Input: part model. Units: mm. Frame: model coordinates. A direction names the side the tool comes from. Give positions to 0.01 mm unless a question says otherwise; leave off trailing zeros. Loops run counter-clockwise (first coordinate to the right, second up) from the corner with the lowest first, then second, coordinate; pieces in that order, holes last. Notation, with made-up numbers: M -26,83 L 16,83 A3 cw 16,88 Z; hole C 86.25,28.25 d9. An arc over 180 degrees is marked long. One line per item, written item: value. Start each with the question number.
(1) Access query for faces 1 (the flat face through (0, 15, -26)), 2 (the flat face through (60, 15, -26)), 3 (the flat face through (30, 23.8, -6)), 4 (the flat face through (-23.293, 32, -27)), 5 (the flat face through (35, 31.5, -34)). Directions: +Z, -Z, +X, -X, +Y, -Y. A direction counts if a zero-diameter tool reaches every point of the face in a straight line with its end or side. Return the directions, or none.
(2) Section C-C on x = -6. Output: boundary loops of the cut face in (y, z), plus the area to 3 significant figures.
(3) Section B-B on z = -18. Output: boundary loops of the cut face in (x, y).
(4) Section A-A on y = 28. Output: boundary loops of the cut face in (x, z) (3 decimals), plus the area to 3 significant figures.
(5) Section D-D on y = 22. Output: boundary loops of the cut face in (x, z) (3 decimals), plus the area to 3 significant figures.
(6) Pull-direction query (Y, two-part tool) for faces 6 (the flat face through (30, 7.4, -6)), 7 (the flat face through (31, 34.5, -27)), 8 (the cylindrical face through (35.243, 15.971, -18.54)); classes: released by +Y, released by -Y, zero draft, split by the parting line, or undercut.
(7) Pin query (flat end, axial travel): P1, Ø1.8, axis at x = 36, z = -36, coming from the +Y side; P2, Ø2.5, axis at x = 26.71, z = -35.54, coming from the +Y side; P3, Ø3.5, axis at x = 69.87, z = -14.16, coming from the -Y side; P4, Ø12, axis at y = 4.5, z = -41.5, coming from the +X side. Return the tip coordinate at first contact, or that it passes through.
(8) Ray query, line 1 along X through (y, z) = (4, -18); line 2 along Y through (x, z) = (10.5, -10); line 3 along X through (y, z) = (13, -20). Return the intervals inside material, ascending. Write a range as from..to.
```python
from build123d import *

# Parameters (mm, degrees)
SKETCH1_W           = 60
SKETCH1_H           = 53.75
BOSS_EXTRUDE1_DEPTH = 29.5
SKETCH2_W           = 110
SKETCH2_H           = 53.75
BOSS_EXTRUDE3_DEPTH = 5
SKETCH3_W           = 12.5
SKETCH3_H           = 16.4
CUT_EXTRUDE1_DEPTH  = 108.691307363
SKETCH4_R           = 1.5
CUT_EXTRUDE2_DEPTH  = 108.691307363
SKETCH7_R           = 3
CUT_EXTRUDE3_DEPTH  = 3
SKETCH8_R           = 1.5
CUT_EXTRUDE4_DEPTH  = 108.691307363
FILLET1_R           = 5


with BuildPart() as part:
    # Sketch1 → Boss-Extrude1 (new body)
    with BuildSketch(Plane(origin=(0, 0, 0), x_dir=(1, 0, 0), z_dir=(0, 1, 0))):
        with Locations((30, 26.875)):
            Rectangle(SKETCH1_W, SKETCH1_H)
    extrude(amount=BOSS_EXTRUDE1_DEPTH)

    # Sketch2 → Boss-Extrude3 (add)
    with BuildSketch(Plane(origin=(0, 29.5, 0), x_dir=(1, 0, 0), z_dir=(0, 1, 0))):
        with Locations((31.707007684, 26.875)):
            Rectangle(SKETCH2_W, SKETCH2_H)
    extrude(amount=BOSS_EXTRUDE3_DEPTH)

    # Sketch3 → Cut-Extrude1 (cut, through all)
    with BuildSketch(Plane.ZY):
        with Locations((-6.25, 15.6)):
            Rectangle(SKETCH3_W, SKETCH3_H)
    extrude(amount=-CUT_EXTRUDE1_DEPTH, mode=Mode.SUBTRACT)

    # Sketch4 → Cut-Extrude2 (cut, through all)
    with BuildSketch(Plane(origin=(0, 34.5, 0), x_dir=(1, 0, 0), z_dir=(0, 1, 0))):
        with Locations(Location((-10.132992316, 14.155, 0), (0, 0, 270))):
            Circle(SKETCH4_R)
        with Locations(Location((69.867007684, 14.155, 0), (0, 0, 270))):
            Circle(SKETCH4_R)
        with Locations(Location((-10.132992316, 44.155, 0), (0, 0, 270))):
            Circle(SKETCH4_R)
        with Locations(Location((69.867007684, 44.155, 0), (0, 0, 270))):
            Circle(SKETCH4_R)
    extrude(amount=-CUT_EXTRUDE2_DEPTH, mode=Mode.SUBTRACT)

    # Sketch7 → Cut-Extrude3 (cut)
    with BuildSketch(Plane(origin=(0, 34.5, 0), x_dir=(1, 0, 0), z_dir=(0, 1, 0))):
        with Locations(Location((41.707007684, 26.875, 0), (0, 0, 270))):
            Circle(SKETCH7_R)
        with Locations(Location((36.707007684, 18.214745962, 0), (0, 0, 270))):
            Circle(SKETCH7_R)
        with Locations(Location((26.707007684, 18.214745962, 0), (0, 0, 270))):
            Circle(SKETCH7_R)
        with Locations(Location((21.707007684, 26.875, 0), (0, 0, 270))):
            Circle(SKETCH7_R)
        with Locations(Location((26.707007684, 35.535254038, 0), (0, 0, 270))):
            Circle(SKETCH7_R)
        with Locations(Location((36.707007684, 35.535254038, 0), (0, 0, 270))):
            Circle(SKETCH7_R)
    extrude(amount=-CUT_EXTRUDE3_DEPTH, mode=Mode.SUBTRACT)

    # Sketch8 → Cut-Extrude4 (cut, through all)
    with BuildSketch(Plane(origin=(0, 34.5, 0), x_dir=(1, 0, 0), z_dir=(0, 1, 0))):
        with Locations(Location((41.707007684, 26.875, 0), (0, 0, 270))):
            Circle(SKETCH8_R)
        with Locations(Location((36.707007684, 18.214745962, 0), (0, 0, 270))):
            Circle(SKETCH8_R)
        with Locations(Location((26.707007684, 18.214745962, 0), (0, 0, 270))):
            Circle(SKETCH8_R)
        with Locations(Location((21.707007684, 26.875, 0), (0, 0, 270))):
            Circle(SKETCH8_R)
        with Locations(Location((26.707007684, 35.535254038, 0), (0, 0, 270))):
            Circle(SKETCH8_R)
        with Locations(Location((36.707007684, 35.535254038, 0), (0, 0, 270))):
            Circle(SKETCH8_R)
    extrude(amount=-CUT_EXTRUDE4_DEPTH, mode=Mode.SUBTRACT)

    # Fillet1
    fillet1_edges = [part.edges().sort_by_distance(p)[0] for p in [
        (-23.292992316, 32, -53.75),
        (-23.292992316, 32, 0),
        (86.707007684, 32, 0),
        (86.707007684, 32, -53.75),
    ]]
    fillet(fillet1_edges, radius=FILLET1_R)


solid = part.part
```
Output values:
1. face 1: +Z, -Z, -X, -Y
1. face 2: +Z, -Z, +X, -Y
1. face 3: +Z, +X, -X
1. face 4: +Z, -Z, -X, +Y, -Y
1. face 5: +Y
2. outline: M 29.5,-53.75 L 34.5,-53.75 L 34.5,0 L 29.5,0 Z
2. area: 269 mm²
3. outline: M -23.29,29.5 L 0,29.5 L 0,0 L 25.22,0 L 25.22,31.5 L 23.71,31.5 L 23.71,34.5 L -23.29,34.5 Z; M 28.19,0 L 35.22,0 L 35.22,31.5 L 33.71,31.5 L 33.71,34.5 L 29.7,34.5 L 29.7,31.5 L 28.19,31.5 Z; M 38.19,0 L 60,0 L 60,29.5 L 86.71,29.5 L 86.71,34.5 L 39.7,34.5 L 39.7,31.5 L 38.19,31.5 Z
4. outline: M 0,-53.75 L 60,-53.75 L 60,0 L 0,0 Z; hole C 21.707,-26.875 d3; hole C 26.707,-35.535 d3; hole C 26.707,-18.215 d3; hole C 36.707,-35.535 d3; hole C 36.707,-18.215 d3; hole C 41.707,-26.875 d3
4. area: 3,180 mm²
5. outline: M 0,-53.75 L 60,-53.75 L 60,-12.5 L 0,-12.5 Z; hole C 21.707,-26.875 d3; hole C 26.707,-35.535 d3; hole C 26.707,-18.215 d3; hole C 36.707,-35.535 d3; hole C 36.707,-18.215 d3; hole C 41.707,-26.875 d3
5. area: 2,430 mm²
6. face 6: undercut
6. face 7: released by +Y
6. face 8: zero draft
7. P1: stops at y = 31.5
7. P2: passes through
7. P3: stops at y = 29.5
7. P4: stops at x = 60
8. line 1: x = 0..25.22, 28.19..35.22, 38.19..60
8. line 2: y = 0..7.4, 23.8..34.5
8. line 3: x = 0..60
